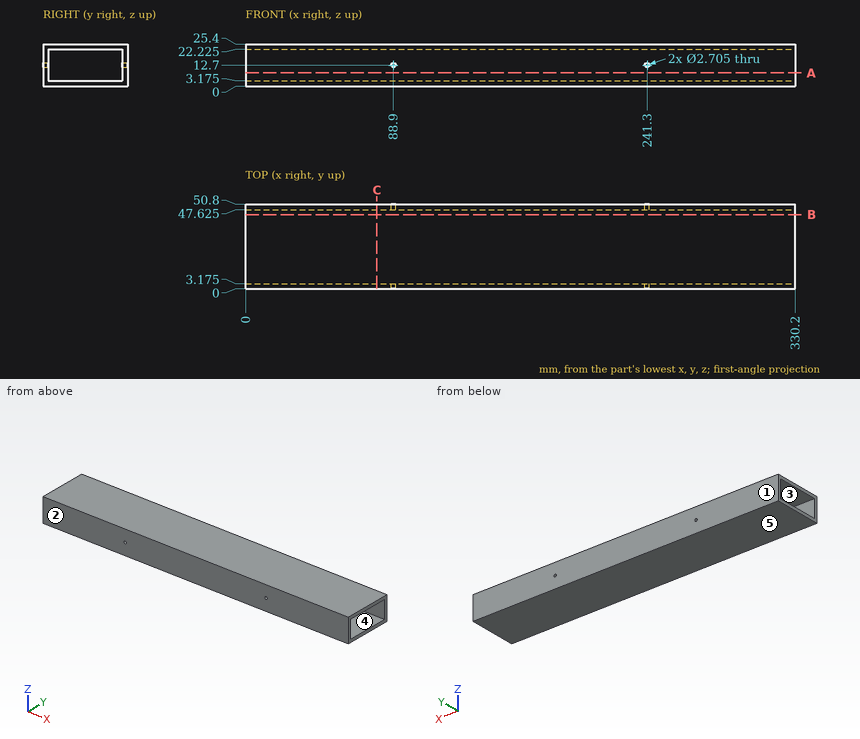
Drawing for the job (mm, zero at the part's lowest x, y, z). A direction names the side the tool comes from. Give positions to 0.01 mm unless a question says otherwise; leave off trailing zeros. Loops run counter-clockwise (first coordinate to the right, second up) from the corner with the lowest first, then second, coordinate; pieces in that order, holes last. Notation, with made-up numbers: (78, 40) - (131, 40) arc R11 ccw to (131, 57) - close; hole circle Ø6 at (9.25, 52.25). An arc over 180 degrees is marked (long way). Write item = value, one per line. Start each with the question number.
1) Probe probe 1 along X at (y, z) = (50, 12.7); probe 2 along Z at (x, y) = (241.3, 2.5); probe 3 along Z at (x, y) = (104.5, 26) (3 decimals). List the from-to ranges inside material, lowest first. Write a range as from..to.
2) Pull direction Y, two halves, no side cores. Call the marked faces 1, 2 and 3: +Y half, -Y half, draft (parallel to the pull), parting line (faces both ways), or undercut.
3) Tool access for the marked faces 4 and 5: list every direction of +Z, -Z, +X, -X, +Y, -Y with a clear straight run to the whole face (end or side of a thin tool).
4) Drop a flat-ended pin along its axis: pin 1 Ø2.5 at (x, z) = (241.3, 12.7) entering from +Y. Give the stop position or say it passes through.
5) Band-saw the part on B-B on y = 44.5. Give the cut face in (x, z) (3 decimals).
6) Band-saw the part on A-A on z = 8. Give the cut face in (x, y) (3 decimals), plus the area to 3 significant figures.
7) Band-saw the part on C-C on x = 79. Give the cut face in (y, z) (3 decimals).
Final values:
q1.probe_1 = 0..87.55, 90.25..239.95, 242.65..330.2
q1.probe_2 = 0..11.35, 14.05..25.4
q1.probe_3 = 0..3.175, 22.225..25.4
q2.face_1 = +Y half
q2.face_2 = -Y half
q2.face_3 = undercut
q3.face_4 = +X, -X
q3.face_5 = -Z, +X, -X, +Y, -Y
q4.pin_1 = through
q5.outline = (0, 0) - (330.2, 0) - (330.2, 3.175) - (0, 3.175) - close; (0, 22.225) - (330.2, 22.225) - (330.2, 25.4) - (0, 25.4) - close
q6.outline = (0, 0) - (330.2, 0) - (330.2, 3.175) - (0, 3.175) - close; (0, 47.625) - (330.2, 47.625) - (330.2, 50.8) - (0, 50.8) - close
q6.area = 2,100 mm²
q7.outline = (0, 0) - (50.8, 0) - (50.8, 25.4) - (0, 25.4) - close; hole (3.175, 3.175) - (47.625, 3.175) - (47.625, 22.225) - (3.175, 22.225) - close
